The listing builds one solid part. Answer for the finished solid, in the listing's coordinates (mm). Face numbers are marked on the shaded views. A direction names the side the tool comes from. Round coordinates to 2 decimals unless told otherwise and drop trailing zeros. Write each loop counter-clockwise with the first axis right and the second up, starting at its lowest first coordinate (ties: lowest second). Pieces come first, ordered by that corner, then holes. Notation, with made-up numbers: (22, 70) - (76, 70) arc R19 cw to (76, 101) - close; hole circle Ø3 at (56.25, 30). An arc over 180 degrees is marked (long way). Answer as CSV lines item,"result". Start each with the question number.
Item 1: A cutting plane is placed at D-D on y = 9.5. Determine the outline of the cut face in (x, z), and give its area (3 significant figures).
Item 2: A cutting plane is placed at C-C on y = 35.5. Determine the outline of the cut face in (x, z), and give its area (3 significant figures).
Item 3: A cutting plane is placed at A-A on x = 0. Determine the outline of the cut face in (y, z), and give its area (3 significant figures).
Item 4: Which of the six approach directions +Z, -Z, +X, -X, +Y, -Y give full straight-line access (tool end or side, diameter ignored) to the marked faces 4 and 5?
Item 5: A cutting plane is placed at B-B on z = 0. Determine the outline of the cut face in (x, y), and give its area (3 significant figures).
Item 6: Straight lines are drawn through the part: line 1 along Y through (x, z) = (0, 1.75); line 2 along Y through (x, z) = (0, 4.75); line 3 along Z through (x, y) = (-3, 16.5). For each, find the intervals that lie inside material, in ascending order. Write a range as [from, to].
Item 7: Flat-ended cylindrical pins translate along their axes: pin 1 (6 mm diameter, centred on x = 0.5, y = 22, fed in from -Z); pin 2 (4 mm diameter, centred on x = -5, y = 21.5, fed in from +Z); pin 3 (4 mm diameter, centred on x = -3.5, y = 25, fed in from -Z); pin 4 (2.5 mm diameter, centred on x = 0, y = 35.5, fed in from -Z) (1 decimal). Find the tip coordinate at first contact, or state that the pin passes through.
Item 8: For a pull along X with two mould halves and no side action, classify the marked faces 1, 2 and 3 as pulls with the +X half, pulls with the -X half, needs draft (parallel to the pull), parting line crosses it, or undercut.
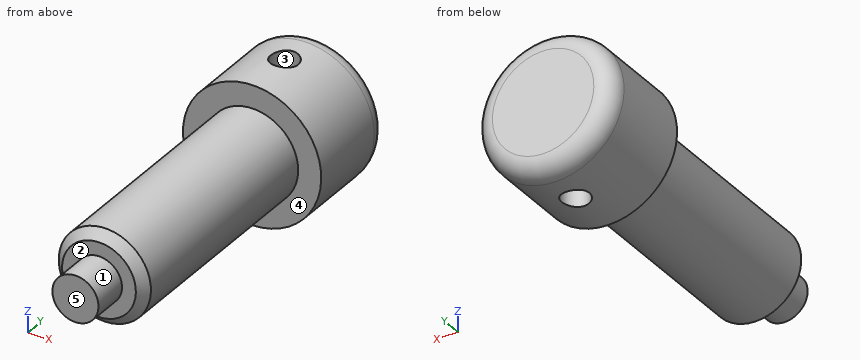
```python
from build123d import *

# Parameters (mm, degrees)
SKETCH_2_W     = 15
SKETCH_2_H     = 1.5
FILLET_1_R     = 2
CHAMFER_1_SIZE = 1


with BuildPart() as part:
    # 草圖1 → 旋轉1 (revolve)
    with BuildSketch(Plane(origin=(0, 0, 0), x_dir=(0, 0, -1), z_dir=(1, 0, 0)), mode=Mode.PRIVATE) as revolve_1_sk:
        Polygon((0, 41), (-7.5, 41), (-7.5, 30), (-5, 30), (-5, 4), (-2.5, 4), (-2.5, 0), (0, 0), align=None)
    revolve(revolve_1_sk.sketch.rotate(Axis((0, 0, 0), (0, 1, 0)), 180), axis=Axis((0, 0, 0), (0, 1, 0)))

    # 草圖2 → 除料-旋轉1 (revolve, cut)
    with BuildSketch(Plane(origin=(0, 0, 0), x_dir=(0, 0, -1), z_dir=(1, 0, 0)), mode=Mode.PRIVATE) as cut_revolve_1_sk:
        with Locations((0, 36.25)):
            Rectangle(SKETCH_2_W, SKETCH_2_H)
    revolve(cut_revolve_1_sk.sketch.rotate(Axis((0, 35.5, 7.5), (0, 0, -1)), 90), axis=Axis((0, 35.5, 7.5), (0, 0, -1)), mode=Mode.SUBTRACT)

    # 圓角1
    fillet_1_edges = [part.edges().sort_by_distance(p)[0] for p in [
        (0, 41, 7.5),
    ]]
    fillet(fillet_1_edges, radius=FILLET_1_R)

    # 導角1
    chamfer_1_edges = [part.edges().sort_by_distance(p)[0] for p in [
        (0, 4, 5),
    ]]
    chamfer(chamfer_1_edges, length=CHAMFER_1_SIZE)


solid = part.part
```
Geometry says:
1,outline,"circle Ø10 at (0, 0)"
1,area,"78.5 mm^2"
2,outline,"(-1.5, -7.35) - (-1.5, 7.35) arc R7.5 ccw to start; (1.5, -7.35) arc R7.5 ccw to (1.5, 7.35) - close"
2,area,"132 mm^2"
3,outline,"(0, -2.5) - (4, -2.5) - (4, -4) - (5, -5) - (30, -5) - (30, -7.5) - (34, -7.5) - (34, 7.5) - (30, 7.5) - (30, 5) - (5, 5) - (4, 4) - (4, 2.5) - (0, 2.5) - close; (37, -7.5) - (39, -7.5) arc R2 ccw to (41, -5.5) - (41, 5.5) arc R2 ccw to (39, 7.5) - (37, 7.5) - close"
3,area,"397 mm^2"
4,face 4,"-Y"
4,face 5,"+Z, -Z, +X, -X, -Y"
5,outline,"(-7.5, 30) - (-5, 30) - (-5, 5) - (-4, 4) - (-2.5, 4) - (-2.5, 0) - (2.5, 0) - (2.5, 4) - (4, 4) - (5, 5) - (5, 30) - (7.5, 30) - (7.5, 39) arc R2 ccw to (5.5, 41) - (-5.5, 41) arc R2 ccw to (-7.5, 39) - close; hole circle Ø3 at (0, 35.5)"
5,area,"435 mm^2"
6,line 1,"y = [0, 34], [37, 41]"
6,line 2,"y = [4.75, 34], [37, 41]"
6,line 3,"z = [-4, 4]"
7,pin 1,"stops at z = -5"
7,pin 2,"stops at z = 4"
7,pin 3,"stops at z = -4.77"
7,pin 4,"passes through"
8,face 1,"parting line crosses it"
8,face 2,"needs draft"
8,face 3,"undercut"
